Source: CAD feature listing. Evaluate the final solid. Frame: model axes, mm. A direction names the side the tool comes from. Round coordinates to 2 decimals unless told otherwise and drop trailing zeros. Loops run counter-clockwise (first coordinate to the right, second up) from the corner with the lowest first, then second, coordinate; pieces in that order, holes last.
(1) Set-up query: faces 1 (the cylindrical face through (9.392, -21.162, 161.177)), 2 (the flat face through (6.35, 2, 2)). Return all of +Z, -Z, +X, -X, +Y, -Y with unobstructed straight access to the full face (end or side cutting, diameter ignored); none if empty.
(2) Mould query, pull axis X, two halves, no side actions, for faces 3 (the cylindrical face through (9.481, 148.997, 46.921)), 4 (the flat face through (0, 2, 2)), 5 (the flat face through (50.8, -79, 114)). Classes: pulls with the +X half, pulls with the -X half, needs draft (parallel to the pull), parting line crosses it, or undercut.
(3) Section A-A, the plane y = 0. Return the cut outline in (x, z), plus the area to 3 significant figures.
(4) First-contact query: pin 1 Ø3 at (x, z) = (27, 120.5) entering from -Y; pin 2 Ø5 at (x, y) = (18.5, -22.5) entering from -Z (3 decimals); pin 3 Ø10 at (y, z) = (73, 127) entering from -X; pin 4 Ø12 at (x, z) = (5.5, 99.5) entering from +Y. Flat tips, straight axial feed; report the tip coordinate or a pass-through.
(5) Section C-C, the plane x = 34.5. Return the cut outline in (y, z), plus the area to 3 significant figures.
(6) Material intervals for probe 1 along X at (y, z) = (104, -101.5); probe 2 along X at (y, z) = (98.5, -129); probe 3 along Y at (x, z) = (8.5, -19.5), sorted ascending.
```python
from build123d import *

# Parameters (mm, degrees)
F0_R     = 162.56
F1_DEPTH = 19.05
F4_DEPTH = 50.8
F7_T     = -6.35


# Not quite as in the source:
# - the program builds the solid bodies; features that only make, move or delete a surface that nothing else refers to are left out


with BuildPart() as f1:
    # F0 (on Right) → F1 (new body)
    with BuildSketch(Plane.YZ):
        Circle(F0_R)
    extrude(amount=F1_DEPTH)

    # F3 (on face) → F4 (join)
    with BuildSketch(Plane(origin=(0, 0, 0), x_dir=(0, -1, 0), z_dir=(-1, 0, 0))):
        with BuildLine():
            ThreePointArc((88.4545554599, 118.760558867), (78.8208582967, 120.384258227), (70.884610199, 114.6868476944))
            ThreePointArc((70.884610199, 114.6868476944), (84.557836343, 95.6406311102), (88.4545554599, 118.760558867))
        make_face()
    extrude(amount=-F4_DEPTH)

    # F7
    f7_openings = [f1.faces().sort_by_distance(p)[0] for p in [
        (50.8, -81.689347, 108.012445),
    ]]
    offset(amount=F7_T, openings=f7_openings, kind=Kind.INTERSECTION)


solid = f1.part
```
Output values:
1. face 1: +X, -X
1. face 2: none
2. face 3: undercut
2. face 4: pulls with the -X half
2. face 5: pulls with the +X half
3. outline: (0, -162.56) - (19.05, -162.56) - (19.05, 162.56) - (0, 162.56) - close; hole (6.35, -156.21) - (12.7, -156.21) - (12.7, 156.21) - (6.35, 156.21) - close
3. area: 4,210 mm2
4. pin 1: stops at y = -88.06
4. pin 2: stops at z = -161.325
4. pin 3: stops at x = 0
4. pin 4: stops at y = 132.98
5. outline: circle Ø25.4 at (-81.69, 108.01); hole circle Ø12.7 at (-81.69, 108.01)
5. area: 380 mm2
6. probe 1: x = 0 to 6.35, 12.7 to 19.05
6. probe 2: x = 0 to 19.05
6. probe 3: y = -161.39 to -154.99, 154.99 to 161.39
